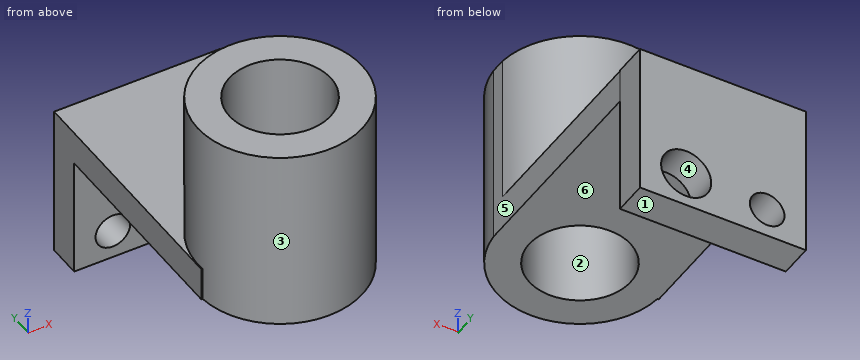
```python
from build123d import *

# Parameters (mm, degrees)
F6_DEPTH  = 25.4
F1_DEPTH  = 254
F7_DEPTH  = 50.8
F8_W      = 249.756782063
F8_H      = 50.8
F2_DEPTH  = 50.8
F9_R      = 26.1205140938
F10_DEPTH = 25.4
F11_DEPTH = 25.4
F3_R      = 37.8459994155
F4_DEPTH  = 558.8


with BuildPart() as f6:
    # F0 (on Top) → F6 (new body)
    with BuildSketch(Plane.XY):
        with BuildLine():
            ThreePointArc((-123.9480513415, 27.3783540638), (0, -85.553869405), (123.9480513415, 27.3783540638))
            Line((123.9480513415, 27.3783540638), (75.5778377526, 27.3783540638))
            ThreePointArc((75.5778377526, 27.3783540638), (0, -37.5243171246), (-75.5778377526, 27.3783540638))
            Line((-75.5778377526, 27.3783540638), (-123.9480513415, 27.3783540638))
        make_face()
        with BuildLine():
            Line((75.5778377526, 27.3783540638), (123.9480513415, 27.3783540638))
            Line((123.9480513415, 27.3783540638), (123.9480513415, 50.4845345108))
            ThreePointArc((123.9480513415, 50.4845345108), (-11.5530902235, 162.8794956288), (-123.9480513415, 27.3783540638))
            Line((-123.9480513415, 27.3783540638), (-75.5778377526, 27.3783540638))
            ThreePointArc((-75.5778377526, 27.3783540638), (-5.7931995405, 115.1674088457), (76.4557614119, 38.9314442873))
            ThreePointArc((76.4557614119, 38.9314442873), (76.2359645584, 33.1382447468), (75.5778377526, 27.3783540638))
        make_face()
    extrude(amount=F6_DEPTH)

    # F1 (add): a face of the model
    f1_faces = [f6.faces().sort_by_distance(p)[0] for p in [
        (120.4308719295, 38.9314442873, 25.4),
    ]]
    extrude(f1_faces, amount=F1_DEPTH)

    # F0 (on Top) → F7 (join)
    with BuildSketch(Plane.XY):
        with BuildLine():
            Line((-125.8087307215, 27.3783540638), (-123.9480513415, 27.3783540638))
            ThreePointArc((-123.9480513415, 27.3783540638), (-11.5530902235, 162.8794956288), (123.9480513415, 50.4845345108))
            Line((123.9480513415, 50.4845345108), (123.9480513415, 350.5234718323))
            Line((123.9480513415, 350.5234718323), (-125.8087307215, 350.5234718323))
            Line((-125.8087307215, 350.5234718323), (-125.8087307215, 27.3783540638))
        make_face()
    extrude(amount=F7_DEPTH)

    # F8 (on face) → F2 (join)
    with BuildSketch(Plane(origin=(0, 350.5234718323, 0), x_dir=(-1, 0, 0), z_dir=(0, 1, 0))):
        Polygon((-123.9480513415, 0), (-123.9480513415, 50.8), (-124.6591806412, 50.8), (-124.6591806412, -182.3397576809), (125.8087307215, -182.3397576809), (125.8087307215, 0), align=None)
        with Locations((0.93033969, 25.4)):
            Rectangle(F8_W, F8_H)
    extrude(amount=F2_DEPTH)

    # F9 (on face) → F10 (cut)
    with BuildSketch(Plane(origin=(0, 401.3234718323, 0), x_dir=(-1, 0, 0), z_dir=(0, 1, 0))):
        with Locations((67.3247128725, -138.6014223099)):
            Circle(F9_R)
    extrude(amount=-F10_DEPTH, mode=Mode.SUBTRACT)

    # F11 (cut): a face of the model
    f11_faces = [f6.faces().sort_by_distance(p)[0] for p in [
        (-67.3247128725, 375.9234718323, -138.6014223099),
    ]]
    extrude(f11_faces, amount=-F11_DEPTH, mode=Mode.SUBTRACT)

    # F3 (on face) → F4 (cut)
    with BuildSketch(Plane(origin=(0, 401.3234718323, 0), x_dir=(-1, 0, 0), z_dir=(0, 1, 0))):
        with Locations((-54.9964085221, -129.5623332262)):
            Circle(F3_R)
    extrude(amount=-F4_DEPTH, mode=Mode.SUBTRACT)


solid = f6.part
```
Can you work these out from the model? Positions are in its coordinate system, mm. Face numbers are marked on the shaded views. A direction names the side the tool comes from. Coordinates: 2 decimals unless noted, no trailing zeros. Write each loop counter-clockwise with the first axis right and the second up, starting at its lowest first coordinate (ties: lowest second). Pieces come first, ordered by that corner, then holes. Notation, with made-up numbers: M 39.5,19.25 L 59.5,19.25 A23 ccw 59.5,28.25 Z; hole C -12.5,8 d9. An arc over 180 degrees is marked long. Write item = value, one per line. Start each with the question number.
Q1. If we section it at D-D, the plane y = 270.5: Write out the boundary of the cut face in (x, z), then the cut area to 3 significant figures.
Q2. If we section it at B-B, the plane x = 43: Write out the boundary of the cut face in (y, z), then the cut area to 3 significant figures.
Q3. On a 3-axis mill with a long thin cutter (end or side, diameter ignored), from which of +Z, -Z, +X, -X, +Y, -Y can I reach the whole of each face in a straight line? I mean the marked faces 4, 5 and 6. Say none if no direction works.
Q4. Thinking about a two-plate mould opening in X: for the marked faces 1, 2 and 3, which applies, released by +X, released by -X, zero draft, split by the parting line, or undercut?
Q5. If we section it at A-A, the plane x = 0: Write out the boundary of the cut face in (y, z), then the cut area to 3 significant figures.
Q6. I'm going to push flat-ended pins straight in: pin 1 (1.5 mm diameter, centred on x = -125, z = 19, fed in from -Y); pin 2 (1.5 mm diameter, centred on x = -34.5, z = 155, fed in from -Y); pin 3 (8 mm diameter, centred on x = 79, y = 246.5, fed in from -Z); pin 4 (4 mm diameter, centred on x = 42.5, z = -98, fed in from +Y). Where does each tip first touch, or does it pass through?
Q7. If I drill on L1, parallel to Y at x = 0.5, z = 100.5; L2, parallel to X at y = 42, z = 180; L3, parallel to Y at x = -78, z = -23.5, over which ranges is the centre line in solid material (lowest first)? Write a range as [from, to].
Q8. If we section it at C-C, the plane z = 25: Write out the boundary of the cut face in (x, y).
Check sheet entries:
q1.outline = M -125.81,0 L 123.95,0 L 123.95,50.8 L -125.81,50.8 Z
q1.area = 12,700 mm²
q2.outline = M -77.89,0 L -24.29,0 L -24.29,279.4 L -77.89,279.4 Z; M 102.15,0 L 350.52,0 L 350.52,-93.67 L 401.32,-93.67 L 401.32,50.8 L 155.75,50.8 L 155.75,279.4 L 102.15,279.4 Z; M 350.52,-182.34 L 401.32,-182.34 L 401.32,-165.46 L 350.52,-165.46 Z
q2.area = 48,000 mm²
q3.face_4 = +Y, -Y
q3.face_5 = +Z, -Z, +X, -Y
q3.face_6 = -Z, +X, -X, -Y
q4.face_1 = zero draft
q4.face_2 = undercut
q4.face_3 = split by the parting line
q5.outline = M -85.55,0 L -37.52,0 L -37.52,279.4 L -85.55,279.4 Z; M 115.39,0 L 350.52,0 L 350.52,-182.34 L 401.32,-182.34 L 401.32,50.8 L 163.42,50.8 L 163.42,279.4 L 115.39,279.4 Z
q5.area = 48,200 mm²
q6.pin_1 = 27.38
q6.pin_2 = -80.89
q6.pin_3 = 0
q6.pin_4 = through
q7.L1 = [-85.55, -37.52], [115.39, 163.42]
q7.L2 = [-124.45, -76.39], [76.39, 123.95]
q7.L3 = [350.52, 401.32]
q8.outline = M -125.81,27.38 L -123.95,27.38 A124.49 ccw 123.95,27.38 L 123.95,350.52 L 124.66,350.52 L 124.66,401.32 L -125.81,401.32 Z; hole C 0,38.93 d152.91
